Work out the finished part from the listing and answer in its coordinate system (mm). A direction names the side the tool comes from. Give positions to 0.01 mm unless a question says otherwise; leave off trailing zeros. Order: outer loops, then holes, each group sorted by start corner. A loop starts at its lowest first (then second) coordinate and runs counter-clockwise, first axis right, second up. Notation, with made-up numbers: (63.5, -22.5) - (100.5, -22.5) arc R16 cw to (100.5, -16.5) - close; hole circle Ø11 at (69.25, 70.5). An arc over 180 degrees is marked (long way). Put each result on its own line as item: value.
```python
from build123d import *

# Parameters (mm, degrees)
BOSS_EXTRUDE1_DEPTH = 2


with BuildPart() as part:
    # Sketch1 → Boss-Extrude1 (new body)
    with BuildSketch(Plane(origin=(0, 0, 0), x_dir=(1, 0, 0), z_dir=(0, 1, 0))):
        Polygon((48.656170244, -59.969878742), (-48.656170244, -59.969878742), (-62.091199086, -73.404907585), (-73.404907585, -62.091199086), (-59.969878742, -48.656170244), (-59.969878742, 48.656170244), (-73.404907585, 62.091199086), (-62.091199086, 73.404907585), (-48.656170244, 59.969878742), (48.656170244, 59.969878742), (62.091199086, 73.404907585), (73.404907585, 62.091199086), (59.969878742, 48.656170244), (59.969878742, -48.656170244), (73.404907585, -62.091199086), (62.091199086, -73.404907585), align=None)
        Polygon((59.050639927, 68.243028082), (68.243028082, 59.050639927), (51.979572115, 42.78718396), (42.78718396, 51.979572115), align=None, mode=Mode.SUBTRACT)
        Polygon((68.243028082, -59.050639927), (51.979572115, -42.78718396), (42.78718396, -51.979572115), (59.050639927, -68.243028082), align=None, mode=Mode.SUBTRACT)
        Polygon((-59.050639927, -68.243028082), (-68.243028082, -59.050639927), (-51.979572115, -42.78718396), (-42.78718396, -51.979572115), align=None, mode=Mode.SUBTRACT)
        Polygon((-68.243028082, 59.050639927), (-51.979572115, 42.78718396), (-42.78718396, 51.979572115), (-59.050639927, 68.243028082), align=None, mode=Mode.SUBTRACT)
    extrude(amount=BOSS_EXTRUDE1_DEPTH)


solid = part.part
```
(1) Determine the mould class of faces 4 (the face through (67.669, 0.986, -67.827)), 5 (the face through (-55.28, 0.986, 66.593)), 6 (the face through (47.448, 0.986, -47.319)) for opening direction Z: pulls with the +Z half, pulls with the -Z half, needs draft (parallel to the pull), parting line crosses it, or undercut.
Geometry check:
face 4: pulls with the -Z half
face 5: pulls with the +Z half
face 6: undercut
(2) Given pin 1 (0.6 mm diameter, centred on y = 1.5, z = -3.5, fed in from -X); pin 2 (1 mm diameter, centred on x = -16, y = 1, fed in from +Z), each flat-ended and moving along its own axis, determine where each tip first touches the part or whether it passes through.
Geometry check:
pin 1: stops at x = -59.97
pin 2: stops at z = 59.97
(3) Section B-B, the plane z = 26 is taken. Write down the section's boundary in (x, y).
Geometry check:
outline: (-59.97, 0) - (59.97, 0) - (59.97, 2) - (-59.97, 2) - close
(4) Straight lines are drawn through the part: line 1 (Z direction, x = 54, y = 0.2); line 2 (Z direction, x = 44, y = 0.25); line 3 (X direction, y = 1.65, z = 24). For each, find the intervals that lie inside material, in ascending order.
Geometry check:
line 1: z = -65.31 to -63.19, -44.81 to 44.81, 63.19 to 65.31
line 2: z = -59.97 to -53.19, -50.77 to 50.77, 53.19 to 59.97
line 3: x = -59.97 to 59.97
(5) A tool of negligible diameter and unlimited length cuts with its end or side. For faces 1 (the face through (47.448, 0.986, 47.319)), 2 (the face through (55.28, 0.986, -66.593)), 3 (the face through (55.468, 0.986, 66.781)), from which of +Z, -Z, +X, -X, +Y, -Y can it reach the whole face along a straight path? Write none if from no direction.
Geometry check:
face 1: +Y, -Y
face 2: -Z, +Y, -Y
face 3: +Z, +Y, -Y
(6) Section C-C, the plane x = -31 is taken. Write down the section's boundary in (y, z).
Geometry check:
outline: (0, -59.97) - (2, -59.97) - (2, 59.97) - (0, 59.97) - close
(7) Section A-A, the plane y = 0.6 is taken. Count the separate pieces of the cut face and the enclosed holes in it, then the cut area to 3 significant figures.
Geometry check:
separate pieces: 1
enclosed holes: 4
area: 14,100 mm²
